from build123d import *

# Parameters (mm, degrees)
SKETCH_1_R          = 9.5
EXTRUDE_1_DEPTH     = 10
SKETCH_2_R          = 8.5
SKETCH_2_R_2        = 9.5
CUT_EXTRUDE_1_DEPTH = 5
SKETCH_3_R          = 3.25
SKETCH_3_R_2        = 2
EXTRUDE_2_DEPTH     = 5
SKETCH_4_W          = 16
SKETCH_4_H          = 2
CUT_EXTRUDE_2_DEPTH = 6


with BuildPart() as part:
    # Эскиз1 → Бобышка-Вытянуть1 (new body)
    with BuildSketch(Plane(origin=(0, 0, 0), x_dir=(1, 0, 0), z_dir=(0, 1, 0))):
        with BuildLine():
            Line((-20, 18), (20, 18))
            ThreePointArc((20, 18), (27.071067812, 15.071067812), (30, 8))
            Line((30, 8), (30, -2))
            ThreePointArc((30, -2), (27.071067812, -9.071067812), (20, -12))
            Line((20, -12), (-20, -12))
            ThreePointArc((-20, -12), (-27.071067812, -9.071067812), (-30, -2))
            Line((-30, -2), (-30, 8))
            ThreePointArc((-30, 8), (-27.071067812, 15.071067812), (-20, 18))
        make_face()
        with Locations((-10, 0)):
            Circle(SKETCH_1_R, mode=Mode.SUBTRACT)
        with Locations((10, 0)):
            Circle(SKETCH_1_R, mode=Mode.SUBTRACT)
    extrude(amount=EXTRUDE_1_DEPTH)

    # Эскиз2 → Вырез-Вытянуть1 (cut)
    with BuildSketch(Plane(origin=(0, 10, 0), x_dir=(1, 0, 0), z_dir=(0, 1, 0))):
        with Locations((-20, -2)):
            Circle(SKETCH_2_R)
        with Locations((-20, 8)):
            Circle(SKETCH_2_R)
        with Locations((-10, 0)):
            Circle(SKETCH_2_R_2)
        with BuildLine():
            Line((20, 16.5), (-20, 16.5))
            ThreePointArc((-20, 16.5), (-14.492370575, 14.474258113), (-11.609926002, 9.362592497))
            ThreePointArc((-11.609926002, 9.362592497), (-3.878084328, 7.26444413), (-0.5, 0))
            ThreePointArc((-0.5, 0), (-5.086783087, -8.13082404), (-14.417957802, -8.410210988))
            ThreePointArc((-14.417957802, -8.410210988), (-17.01979811, -9.960426917), (-20, -10.5))
            Line((-20, -10.5), (20, -10.5))
            ThreePointArc((20, -10.5), (17.01979811, -9.960426917), (14.417957802, -8.410210988))
            ThreePointArc((14.417957802, -8.410210988), (0.616398255, -1.48257151), (11.609926002, 9.362592497))
            ThreePointArc((11.609926002, 9.362592497), (14.492370575, 14.474258113), (20, 16.5))
        make_face()
        with BuildLine():
            ThreePointArc((-26.873863542, 3), (-28.08324935, 5.371106707), (-28.5, 8))
            Line((-28.5, 8), (-28.5, -2))
            ThreePointArc((-28.5, -2), (-28.08324935, 0.628893293), (-26.873863542, 3))
        make_face()
        with Locations((20, -2)):
            Circle(SKETCH_2_R)
        with Locations((20, 8)):
            Circle(SKETCH_2_R)
        with Locations((10, 0)):
            Circle(SKETCH_2_R_2)
        with BuildLine():
            Line((28.5, -2), (28.5, 8))
            ThreePointArc((28.5, 8), (28.08324935, 5.371106707), (26.873863542, 3))
            ThreePointArc((26.873863542, 3), (28.08324935, 0.628893293), (28.5, -2))
        make_face()
    extrude(amount=-CUT_EXTRUDE_1_DEPTH, mode=Mode.SUBTRACT)

    # Эскиз3 → Бобышка-Вытянуть2 (add)
    with BuildSketch(Plane(origin=(0, 5, 0), x_dir=(1, 0, 0), z_dir=(0, 1, 0))):
        with Locations((-23.5, 3)):
            Circle(SKETCH_3_R)
        with Locations((-23.5, 3)):
            Circle(SKETCH_3_R_2, mode=Mode.SUBTRACT)
        with Locations((23.5, 3)):
            Circle(SKETCH_3_R)
        with Locations((23.5, 3)):
            Circle(SKETCH_3_R_2, mode=Mode.SUBTRACT)
    extrude(amount=EXTRUDE_2_DEPTH)

    # Эскиз4 → Вырез-Вытянуть2 (cut, through all)
    with BuildSketch(Plane(origin=(0, 5, 0), x_dir=(1, 0, 0), z_dir=(0, 1, 0))):
        with Locations((0, 14)):
            Rectangle(SKETCH_4_W, SKETCH_4_H)
    extrude(amount=-CUT_EXTRUDE_2_DEPTH, mode=Mode.SUBTRACT)


solid = part.part
Could you check a few things on this model? Use its own coordinates, in mm. A direction names the side the tool comes from. Round coordinates to 2 decimals unless told otherwise and drop trailing zeros. Order: outer loops, then holes, each group sorted by start corner. A loop starts at its lowest first (then second) coordinate and runs counter-clockwise, first axis right, second up. Notation, with made-up numbers: M 43,-32.75 L 95,-32.75 A24 cw 95,-6.75 Z; hole C 13.25,-37.75 d3. An arc over 180 degrees is marked long. One line per item, written item: value.
(1) Imagine slicing it at D-D (z = 3.5). Write out the boundary of the cut face in (x, y), and give its area (3 significant figures).
Ans:
outline: M -29.89,0 L -18.83,0 L -18.83,5 L -28.37,5 L -28.37,10 L -29.89,10 Z; M -1.17,0 L 1.17,0 L 1.17,5 L -1.17,5 Z; M 18.83,0 L 29.89,0 L 29.89,10 L 28.37,10 L 28.37,5 L 18.83,5 Z
area: 137 mm^2
(2) Imagine slicing it at C-C (y = 3). Write out the boundary of the cut face in (x, z).
Ans:
outline: M -30,-8 A10 ccw -20,-18 L 20,-18 A10 ccw 30,-8 L 30,2 A10 ccw 20,12 L -20,12 A10 ccw -30,2 Z; hole C -10,0 d19; hole M -8,-15 L 8,-15 L 8,-13 L -8,-13 Z; hole C 10,0 d19
(3) Which directions (+Z, -Z, +X, -X, +Y, -Y) give clear straight access to the entire face, cutting with the end or side of a thin tool? Please do faces 4 (the cylindrical face through (-25.1, 7.5, -1.8)), 5 (the flat face through (0, 5, 12)), 6 (the flat face through (8, 3, -14)).
Ans:
face 4: +Y
face 5: +Z, +X, -X, +Y, -Y
face 6: +Y, -Y
(4) If we mould it in two halves opening along Z, with no side actions, what happens to faces 1 (the flat face through (0.1, 10, -17.5)), 2 (the flat face through (0, 8, -16.5)), 3 (the cylindrical face through (-26.99, 4.93, 9.15))? For each: released by +Z, released by -Z, zero draft, split by the parting line, or undercut.
Ans:
face 1: zero draft
face 2: undercut
face 3: released by +Z
(5) Imagine slicing it at B-B (x = -10). Write out the boundary of the cut face in (y, z).
Ans:
outline: M 0,-18 L 10,-18 L 10,-16.5 L 5,-16.5 L 5,-9.5 L 0,-9.5 Z; M 0,9.5 L 5,9.5 L 5,10.5 L 10,10.5 L 10,12 L 0,12 Z
(6) I need wall thicknesses on line 1 along X through (y, z) = (6.2, -3); line 2 along X through (y, z) = (0.5, 0.5); line 3 along X through (y, z) = (2.25, 8.75). Which ranges of each line are inside material? Lowest first, please. Write a range as from..to.
Ans:
line 1: x = -30..-28.5, -26.75..-25.5, -21.5..-20.25, 20.25..21.5, 25.5..26.75, 28.5..30
line 2: x = -30..-19.49, -0.51..0.51, 19.49..30
line 3: x = -27.38..-13.7, -6.3..6.3, 13.7..27.38
(7) Imagine slicing it at A-A (y = 6.75). Write out the boundary of the cut face in (x, z), and give its area (3 significant figures).
Ans:
outline: M -30,-8 A10 ccw -20,-18 L 20,-18 A10 ccw 30,-8 L 30,2 A10 ccw 20,12 L -20,12 A10 ccw -30,2 Z; C -23.5,-3 d6.5; C 23.5,-3 d6.5; hole M -28.5,-8 A8.5 ccw -20,-16.5 L 20,-16.5 A8.5 ccw 28.5,-8 L 28.5,2 A8.5 ccw 20,10.5 L -20,10.5 A8.5 ccw -28.5,2 Z; hole C -23.5,-3 d4; hole C 23.5,-3 d4
area: 278 mm^2
(8) I'm going to push flat-ended pins straight in: P1, Ø13.5, axis at x = 6.5, z = -1, coming from the +Y side; P2, Ø5, axis at y = 8.5, z = 8, coming from the +X side; P3, Ø0.6, axis at y = 2, z = -13.5, coming from the -X side. Where does each tip first touch, or does it pass through?
Ans:
P1: stops at y = 5
P2: stops at x = 29.37
P3: stops at x = -28.54
